Source: CAD feature listing. Evaluate the final solid. Frame: model axes, mm. Face numbers are marked on the shaded views. A direction names the side the tool comes from. Coordinates: 2 decimals unless noted, no trailing zeros. Write each loop counter-clockwise with the first axis right and the second up, starting at its lowest first coordinate (ties: lowest second). Pieces come first, ordered by that corner, then holes. Notation, with made-up numbers: M 13,-12.5 L 21,-12.5 A17 ccw 21,15.5 Z; hole C 31,36.5 d3. An arc over 180 degrees is marked long. Answer as CSV lines item,"result". Start each with the question number.
1. Mould query, pull axis Z, two halves, no side actions, for the marked faces 6, 7, 8 and 9. Classes: pulls with the +Z half, pulls with the -Z half, needs draft (parallel to the pull), parting line crosses it, or undercut.
2. Line query: probe 1 along Z at (x, y) = (4, 9.25); probe 2 along X at (y, z) = (4.75, -4.5); probe 3 along X at (y, z) = (4, -10). Output: solid intervals per line, ascending. Write a range as [from, to].
3. Section B-B on x = -13.95. Return the cut outline in (y, z).
4. Section D-D on x = 4.5. Return the cut outline in (y, z).
5. Reachability of the marked faces 1, 2, 3, 4 and 5 from +Z, -Z, +X, -X, +Y, -Y: full face, straight path, thin tool, end or side. Return the list, or none.
6. Section C-C on z = 11. Return the cut outline in (x, y), plus the area to 3 significant figures.
7. Contact query for flat-ended pins moving along their axis: pin 1 Ø0.6 at (x, y) = (14, 8) entering from +Z; pin 2 Ø5.5 at (y, z) = (4, -17) entering from -X; pin 3 Ø1 at (x, z) = (-4, -9) entering from +Y. Output: stop coordinate, or through.
8. Section A-A on y = 3.25. Return the cut outline in (x, z).
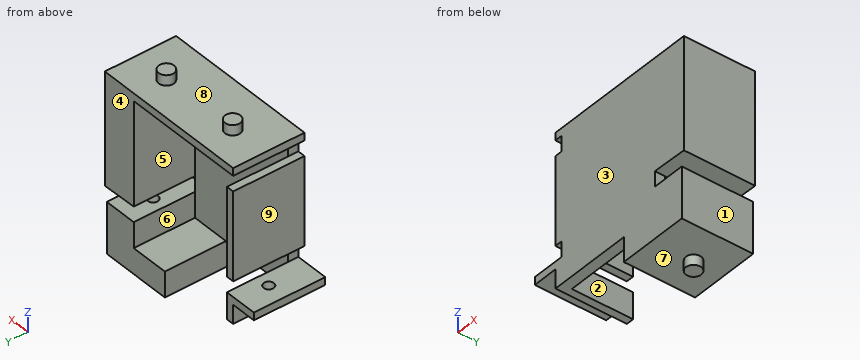
```python
from build123d import *

# Parameters (mm, degrees)
SKETCH_1_W          = 22.5
SKETCH_1_H          = 30
EXTRUDE_1_DEPTH     = 2
SKETCH_2_W          = 22.5
SKETCH_2_H          = 1.5
EXTRUDE_2_DEPTH     = 12
EXTRUDE_4_REACH     = 25.4
SKETCH_3_W          = 1.5
SKETCH_3_H          = 17.3
SKETCH_3_H_2        = 1.5
SKETCH_6_R          = 1.5
EXTRUDE_5_DEPTH     = 2
EXTRUDE_START       = 2
SKETCH_7_R          = 1.5
EXTRUDE_6_DEPTH     = 2
CUT_EXTRUDE_1_REACH = 38.469
SKETCH_8_R          = 1


with BuildPart() as part:
    # 草图1 → 凸台-拉伸1 (new body)
    with BuildSketch(Plane(origin=(0, 0, 0), x_dir=(1, 0, 0), z_dir=(0, 1, 0))):
        Rectangle(SKETCH_1_W, SKETCH_1_H)
    extrude(amount=EXTRUDE_1_DEPTH)

    # 草图2 → 凸台-拉伸2 (add)
    with BuildSketch(Plane(origin=(0, 2, 0), x_dir=(1, 0, 0), z_dir=(0, 1, 0))):
        with Locations((0, -14.25)):
            Rectangle(SKETCH_2_W, SKETCH_2_H)
    extrude(amount=EXTRUDE_2_DEPTH)

    # 凸台-拉伸4: up to this face of the body (flat: up to its plane)
    extrude_4_end = Plane(part.part.faces().sort_by_distance((0, 14, 14.25))[0])
    # 草图3 → 凸台-拉伸4 (add, up to the picked face)
    with BuildSketch(Plane.XZ, mode=Mode.PRIVATE) as extrude_4_sk1:
        Polygon((-11.25, -15), (-12.75, -15), (-12.75, -11.3), (-17.75, -11.3), (-17.75, -9.8), (-12.75, -9.8), (-11.25, -9.8), align=None)
    extrude_4_tool1 = split(extrude(extrude_4_sk1.sketch, amount=-EXTRUDE_4_REACH, mode=Mode.PRIVATE), bisect_by=extrude_4_end, keep=Keep.BOTH, mode=Mode.PRIVATE)
    # 草图3 → 凸台-拉伸4 (add, up to the picked face)
    with BuildSketch(Plane.XZ, mode=Mode.PRIVATE) as extrude_4_sk2:
        with Locations((-12, 1.85)):
            Rectangle(SKETCH_3_W, SKETCH_3_H)
    extrude_4_tool2 = split(extrude(extrude_4_sk2.sketch, amount=-EXTRUDE_4_REACH, mode=Mode.PRIVATE), bisect_by=extrude_4_end, keep=Keep.BOTH, mode=Mode.PRIVATE)
    # 草图3 → 凸台-拉伸4 (add, up to the picked face)
    with BuildSketch(Plane.XZ, mode=Mode.PRIVATE) as extrude_4_sk3:
        with Locations((-12, 14.25)):
            Rectangle(SKETCH_3_W, SKETCH_3_H_2)
    extrude_4_tool3 = split(extrude(extrude_4_sk3.sketch, amount=-EXTRUDE_4_REACH, mode=Mode.PRIVATE), bisect_by=extrude_4_end, keep=Keep.BOTH, mode=Mode.PRIVATE)
    # 草图3 → 凸台-拉伸4 (add, up to the picked face)
    with BuildSketch(Plane.XZ, mode=Mode.PRIVATE) as extrude_4_sk4:
        Polygon((11.25, -9.8), (11.25, -14.8), (3.75, -14.8), (3.75, -19.8), (17.75, -19.8), (17.75, -11.3), (17.75, -9.8), (12.75, -9.8), align=None)
    extrude_4_tool4 = split(extrude(extrude_4_sk4.sketch, amount=-EXTRUDE_4_REACH, mode=Mode.PRIVATE), bisect_by=extrude_4_end, keep=Keep.BOTH, mode=Mode.PRIVATE)
    # 草图3 → 凸台-拉伸4 (add, up to the picked face)
    with BuildSketch(Plane.XZ, mode=Mode.PRIVATE) as extrude_4_sk5:
        Polygon((18.25, -7), (11.25, -6.8), (11.25, 15), (18.25, 15), align=None)
    extrude_4_tool5 = split(extrude(extrude_4_sk5.sketch, amount=-EXTRUDE_4_REACH, mode=Mode.PRIVATE), bisect_by=extrude_4_end, keep=Keep.BOTH, mode=Mode.PRIVATE)
    add(extrude_4_tool1.solids().sort_by(Axis((-12, 0, -14.916759), (0, 1, 0)))[0])
    add(extrude_4_tool2.solids().sort_by(Axis((-12, 0, 1.85), (0, 1, 0)))[0])
    add(extrude_4_tool3.solids().sort_by(Axis((-12, 0, 14.25), (0, 1, 0)))[0])
    add(extrude_4_tool4.solids().sort_by(Axis((11.939024, 0, -15.714634), (0, 1, 0)))[0])
    add(extrude_4_tool5.solids().sort_by(Axis((14.755327, 0, 4.049924), (0, 1, 0)))[0])

    # 草图6 → 凸台-拉伸5 (add)
    with BuildSketch(Plane(origin=(0, 0, -19.8), x_dir=(-1, 0, 0), z_dir=(0, 0, -1))):
        with Locations((-10.75, 8)):
            Circle(SKETCH_6_R)
    extrude(amount=EXTRUDE_5_DEPTH)

    # 草图7 → 凸台-拉伸6 (add)
    with BuildSketch(Plane.XY.offset(15).offset(EXTRUDE_START)):
        with Locations(Location((10.75, 8, 0), (0, 0, 180))):
            Circle(SKETCH_7_R)
        with Locations(Location((-5.25, 8, 0), (0, 0, 180))):
            Circle(SKETCH_7_R)
    extrude(amount=-EXTRUDE_6_DEPTH)

    # 草图8 → 切除-拉伸1 (cut, up to next)
    with BuildSketch(Plane(origin=(0, 0, -11.3), x_dir=(-1, 0, 0), z_dir=(0, 0, -1)), mode=Mode.PRIVATE) as cut_extrude_1_sk1:
        with Locations((13.95, 8)):
            Circle(SKETCH_8_R)
    cut_extrude_1_tool1 = extrude(cut_extrude_1_sk1.sketch, amount=-CUT_EXTRUDE_1_REACH, mode=Mode.PRIVATE) & part.part
    # 草图8 → 切除-拉伸1 (cut, up to next)
    with BuildSketch(Plane(origin=(0, 0, -11.3), x_dir=(-1, 0, 0), z_dir=(0, 0, -1)), mode=Mode.PRIVATE) as cut_extrude_1_sk2:
        with Locations(Location((-13.95, 8, 0), (0, 0, 180))):
            Circle(SKETCH_8_R)
    cut_extrude_1_tool2 = extrude(cut_extrude_1_sk2.sketch, amount=-CUT_EXTRUDE_1_REACH, mode=Mode.PRIVATE) & part.part
    add(cut_extrude_1_tool1.solids().sort_by_distance((-13.95, 8, -11.3))[0], mode=Mode.SUBTRACT)
    add(cut_extrude_1_tool2.solids().sort_by_distance((13.95, 8, -11.3))[0], mode=Mode.SUBTRACT)


solid = part.part
```
Values:
1,face 6,"undercut"
1,face 7,"pulls with the -Z half"
1,face 8,"pulls with the +Z half"
1,face 9,"needs draft"
2,probe 1,"[-19.8, -14.8], [13.5, 15]"
2,probe 2,"[-12.75, -11.25], [11.25, 18.25]"
2,probe 3,"[-17.75, -11.25], [11.25, 17.75]"
3,outline,"M 0,-11.3 L 7,-11.3 L 7,-9.8 L 0,-9.8 Z; M 9,-11.3 L 14,-11.3 L 14,-9.8 L 9,-9.8 Z"
4,outline,"M 0,-19.8 L 14,-19.8 L 14,-14.8 L 2,-14.8 L 2,13.5 L 14,13.5 L 14,15 L 0,15 Z"
5,face 1,"-Z, +X, +Y, -Y"
5,face 2,"-Z, +Y"
5,face 3,"+Z, -Z, +X, -X, -Y"
5,face 4,"+Z, -Z, +X, -X, +Y"
5,face 5,"+Y"
6,outline,"M -11.25,0 L 18.25,0 L 18.25,14 L 11.25,14 L 11.25,2 L -11.25,2 Z"
6,area,"143 mm²"
7,pin 1,"z = 15"
7,pin 2,"x = -12.75"
7,pin 3,"y = 2"
8,outline,"M -17.75,-11.3 L -12.75,-11.3 L -12.75,-15 L -11.25,-15 L -11.25,-9.8 L -17.75,-9.8 Z; M -12.75,-6.8 L -11.25,-6.8 L -11.25,10.5 L -12.75,10.5 Z; M -12.75,13.5 L 11.25,13.5 L 11.25,-6.8 L 18.25,-7 L 18.25,15 L -12.75,15 Z; M 3.75,-19.8 L 17.75,-19.8 L 17.75,-9.8 L 11.25,-9.8 L 11.25,-14.8 L 3.75,-14.8 Z"
